Input: part model. Units: mm. Frame: model coordinates. A direction names the side the tool comes from. Round coordinates to 2 decimals unless told otherwise and drop trailing zeros. Loops run counter-clockwise (first coordinate to the right, second up) from the corner with the lowest first, then second, coordinate; pieces in that order, holes last. Notation, with made-up numbers: M 31.5,33 L 38.5,33 A28 cw 38.5,71 Z; hole C 78,54.5 d7. An arc over 180 degrees is marked long. Use one line per item in the form item = value. Start each with the question number.
Q1. First-contact query: P1, Ø8, axis at x = 25.5, y = 29.5, coming from the -Z side; P2, Ø3, axis at x = 42.5, z = -6, coming from the +Y side (3 decimals). Flat tips, straight axial feed; report the tip coordinate or a pass-through.
Q2. Section query A-A, the plane y = 32. Output: boundary loops of the cut face in (x, z).
Q3. Section query C-C, the plane x = 13. Output: boundary loops of the cut face in (y, z).
Q4. Section query B-B, the plane z = -18. Output: boundary loops of the cut face in (x, y).
Q5. Mould query, pull axis X, two halves, no side actions, for faces 4 (the cylindrical face through (14.77, 11.5, -14.79)), 5 (the flat face through (35, 25, -25)), 6 (the cylindrical face through (56, 13, -15)), 7 (the flat face through (70, 17, -15)). Classes: pulls with the +X half, pulls with the -X half, needs draft (parallel to the pull), parting line crosses it, or undercut.
Q6. Ray query, line 1 along X through (y, z) = (6, -23); line 2 along X through (y, z) = (12, -7.5); line 3 along Y through (x, z) = (10, -15.5). Return the intervals inside material, ascending.
Q7. Access query for faces 1 (the flat face through (35, 0, -15)), 2 (the flat face through (25, 26, -8)), 3 (the flat face through (57, 30, -20)). Directions: +Z, -Z, +X, -X, +Y, -Y. A direction counts if a zero-diameter tool reaches every point of the face in a straight line with its end or side. Return the directions, or none.
Q8. Section query D-D, the plane y = 8. Output: boundary loops of the cut face in (x, z).
```python
from build123d import *

# Parameters (mm, degrees)
SKETCH1_W           = 35
SKETCH1_H           = 30
BOSS_EXTRUDE1_DEPTH = 35
SKETCH2_W           = 35
SKETCH2_H           = 10
CUT_EXTRUDE1_DEPTH  = 10
CUT_EXTRUDE3_DEPTH  = 16.617376189
CUT_EXTRUDE4_DEPTH  = 21
CUT_EXTRUDE5_DEPTH  = 19
SKETCH13_R          = 5
CUT_EXTRUDE6_DEPTH  = 31
SKETCH14_R          = 5
CUT_EXTRUDE7_DEPTH  = 31


with BuildPart() as part:
    # Sketch1 → Boss-Extrude1 (new body)
    with BuildSketch(Plane(origin=(0, 0, 0), x_dir=(1, 0, 0), z_dir=(0, 1, 0))):
        with Locations((17.5, 15)):
            Rectangle(SKETCH1_W, SKETCH1_H)
    boss_extrude1 = extrude(amount=BOSS_EXTRUDE1_DEPTH)

    # Sketch2 → Cut-Extrude1 (cut)
    with BuildSketch(Plane(origin=(0, 35, 0), x_dir=(1, 0, 0), z_dir=(0, 1, 0))):
        with Locations((17.5, 25)):
            Rectangle(SKETCH2_W, SKETCH2_H)
    cut_extrude1 = extrude(amount=-CUT_EXTRUDE1_DEPTH, mode=Mode.SUBTRACT)

    # Sketch8 → Cut-Extrude3 (cut, through all)
    with BuildSketch(Plane(origin=(17.56097561, 17.56097561, 13.170731707), x_dir=(0.780868809, -0.499756038, -0.374817029), z_dir=(0.624695048, 0.624695048, 0.468521286))):
        Polygon((-9.682773237, 21), (22.33284795, 6), (22.33284795, 31), (9.526599475, 37), align=None)
    cut_extrude3 = extrude(amount=CUT_EXTRUDE3_DEPTH, mode=Mode.SUBTRACT)

    # Sketch10 → Cut-Extrude4 (cut, through all)
    with BuildSketch(Plane(origin=(0, 0, -20), x_dir=(-1, 0, 0), z_dir=(0, 0, -1))):
        Polygon((-35, 35), (-25, 35), (-35, 25), align=None)
    extrude(amount=-CUT_EXTRUDE4_DEPTH, mode=Mode.SUBTRACT)

    # Mirror5: Boss-Extrude1, Cut-Extrude1, Cut-Extrude3 across plane
    add(boss_extrude1.mirror(Plane(origin=(35, 35, 0), x_dir=(0, 0, 1), z_dir=(-1, 0, 0))))
    add(cut_extrude1.mirror(Plane(origin=(35, 35, 0), x_dir=(0, 0, 1), z_dir=(-1, 0, 0))), mode=Mode.SUBTRACT)
    add(cut_extrude3.mirror(Plane(origin=(35, 35, 0), x_dir=(0, 0, 1), z_dir=(-1, 0, 0))), mode=Mode.SUBTRACT)

    # Sketch12 → Cut-Extrude5 (cut)
    with BuildSketch(Plane(origin=(0, 0, -20), x_dir=(-1, 0, 0), z_dir=(0, 0, -1))):
        Polygon((-45, 35), (-35, 25), (-35, 35), align=None)
    extrude(amount=-CUT_EXTRUDE5_DEPTH, mode=Mode.SUBTRACT)

    # Sketch13 → Cut-Extrude6 (cut, through all)
    with BuildSketch(Plane.XY):
        with Locations((10, 10)):
            Circle(SKETCH13_R)
    extrude(amount=-CUT_EXTRUDE6_DEPTH, mode=Mode.SUBTRACT)

    # Sketch14 → Cut-Extrude7 (cut, through all)
    with BuildSketch(Plane.XY):
        with Locations((60, 10)):
            Circle(SKETCH14_R)
    extrude(amount=-CUT_EXTRUDE7_DEPTH, mode=Mode.SUBTRACT)


solid = part.part
```
Results found:
q1.P1 = -20
q1.P2 = 23.875
q2.outline = M 0,-20 L 28,-20 L 13,0 L 0,0 Z; M 42,-20 L 70,-20 L 70,0 L 57,0 Z
q3.outline = M 0,-30 L 6,-30 L 6,0 L 0,0 Z; M 14,-30 L 25,-30 L 25,-20 L 35,-20 L 35,-4 L 32,0 L 14,0 Z
q4.outline = M 0,0 L 70,0 L 70,35 L 46.5,35 L 35,23.5 L 23.5,35 L 0,35 Z; hole C 10,10 d10; hole C 60,10 d10
q5.face_4 = undercut
q5.face_5 = needs draft
q5.face_6 = undercut
q5.face_7 = pulls with the +X half
q6.line_1 = 0 to 7, 13 to 57, 63 to 70
q6.line_2 = 0 to 5.42, 14.58 to 55.42, 64.58 to 70
q6.line_3 = 0 to 5, 15 to 35
q7.face_1 = +Z, -Z, +X, -X, -Y
q7.face_2 = +Z, +Y
q7.face_3 = -Z, +X, -X, +Y
q8.outline = M 0,-30 L 5.42,-30 L 5.42,0 L 0,0 Z; M 14.58,-30 L 55.42,-30 L 55.42,0 L 14.58,0 Z; M 64.58,-30 L 70,-30 L 70,0 L 64.58,0 Z
